Print and shaded views of the part. All mm, measured from the part's lowest x, y and z. A direction names the side the tool comes from. Give positions to 0.01 mm unless a question says otherwise; leave off trailing zeros. Loops run counter-clockwise (first coordinate to the right, second up) from the corner with the lowest first, then second, coordinate; pieces in that order, holes last.
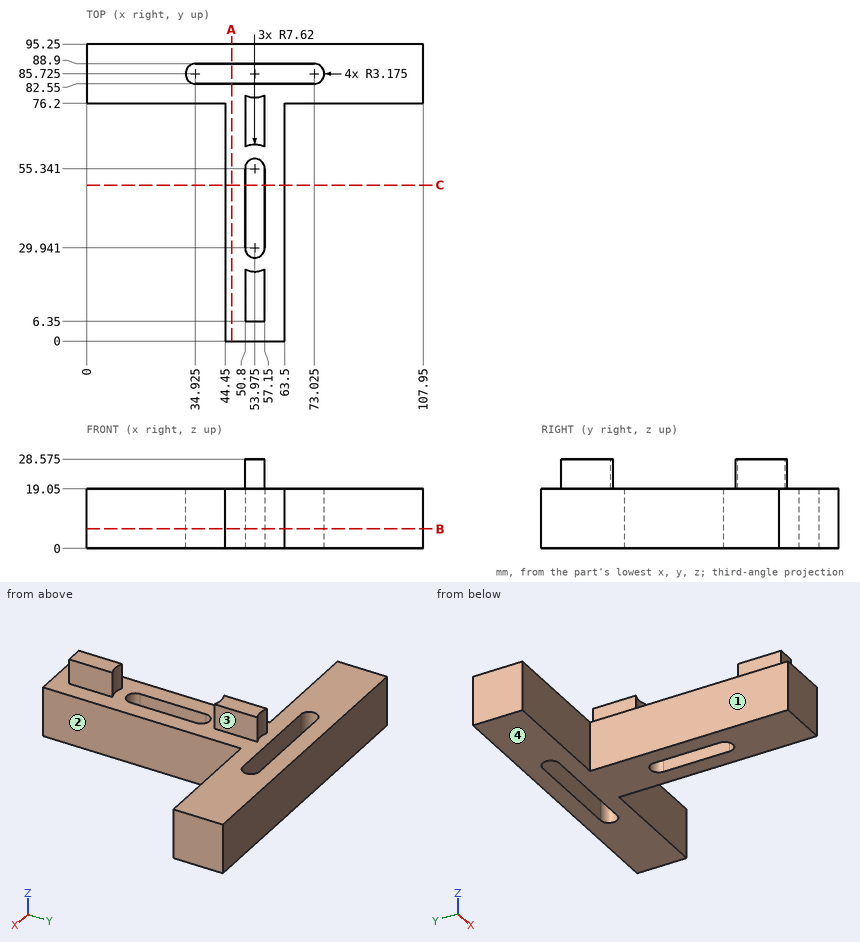
1. Saw through at B-B, the plane z = 6.25. Count the separate pieces of the cut face and the enclosed holes in it, and give its area (3 significant figures).
Responses:
separate pieces: 1
enclosed holes: 2
area: 3,040 mm2
2. Drop flat-ended pins along their axis: pin 1 (1 mm diameter, centred on y = 40.5, z = 10, fed in from -X); pin 2 (7.5 mm diameter, centred on y = 16, z = 24.5, fed in from -X); pin 3 (4 mm diameter, centred on x = 43, y = 21.5, fed in from +Z). Give the stop position or say it passes through.
Responses:
pin 1: stops at x = 44.45
pin 2: stops at x = 50.8
pin 3: stops at z = 19.05
3. Tool access for the marked faces 1, 2, 3 and 4: list every direction of +Z, -Z, +X, -X, +Y, -Y with a clear straight run to the whole face (end or side of a thin tool).
Responses:
face 1: +Z, -Z, -X, -Y
face 2: +Z, -Z, +X, -Y
face 3: +Z, +X, +Y, -Y
face 4: -Z, +X, -X, +Y, -Y
4. Probe line 1 along Y through (x, z) = (46.5, 3.75); line 2 along X through (y, z) = (34, 10); line 3 along Y through (x, z) = (68, 7.5). List the from-to ranges inside material, lowest first.
Responses:
line 1: y = 0 to 82.55, 88.9 to 95.25
line 2: x = 44.45 to 50.8, 57.15 to 63.5
line 3: y = 76.2 to 82.55, 88.9 to 95.25
5. Saw through at C-C, the plane y = 50. List the corners of the cut face in (x, z), and give its area (3 significant figures).
Responses:
outline: (44.45, 0) - (50.8, 0) - (50.8, 19.05) - (44.45, 19.05) - close; (57.15, 0) - (63.5, 0) - (63.5, 19.05) - (57.15, 19.05) - close
area: 242 mm2
6. Saw through at A-A, the plane x = 46.5. List the corners of the cut face in (y, z), and give its area (3 significant figures).
Responses:
outline: (0, 0) - (82.55, 0) - (82.55, 19.05) - (0, 19.05) - close; (88.9, 0) - (95.25, 0) - (95.25, 19.05) - (88.9, 19.05) - close
area: 1,690 mm2
